from build123d import *

# Parameters (mm, degrees)
EXTRUDE_1_DEPTH = 815
SHELL_1_T       = -3


with BuildPart() as part:
    # Эскиз1 → Бобышка-Вытянуть1 (new, symmetric)
    with BuildSketch(Plane.XY):
        with BuildLine():
            Line((-25, -30), (25, -30))
            ThreePointArc((25, -30), (28.535533906, -28.535533906), (30, -25))
            Line((30, -25), (30, 25))
            ThreePointArc((30, 25), (28.535533906, 28.535533906), (25, 30))
            Line((25, 30), (-25, 30))
            ThreePointArc((-25, 30), (-28.535533906, 28.535533906), (-30, 25))
            Line((-30, 25), (-30, -25))
            ThreePointArc((-30, -25), (-28.535533906, -28.535533906), (-25, -30))
        make_face()
    extrude(amount=EXTRUDE_1_DEPTH, both=True)

    # Оболочка1
    shell_1_openings = [part.faces().sort_by_distance(p)[0] for p in [
        (0, 0, 815),
        (0, 0, -815),
    ]]
    offset(amount=SHELL_1_T, openings=shell_1_openings, kind=Kind.INTERSECTION)


solid = part.part
Input: part model. Units: mm. Frame: model coordinates. A direction names the side the tool comes from. Give positions to 0.01 mm unless a question says otherwise; leave off trailing zeros. Write each loop counter-clockwise with the first axis right and the second up, starting at its lowest first coordinate (ties: lowest second). Pieces come first, ordered by that corner, then holes. Notation, with made-up numbers: (-0.5, -3) -> (50.5, -3) arc R12 ccw to (50.5, 4) -> close; hole circle Ø8 at (48, 45.25). An arc over 180 degrees is marked (long way). Use one line per item in the form item = value. Start each with the question number.
1) Section query A-A on x = 5. Return the cut outline in (y, z), then the cut area to 3 significant figures.
2) Set-up query: faces 4 (the flat face through (27, 0, 11)), 5 (the flat face through (-2, -29, -815)). Return all of +Z, -Z, +X, -X, +Y, -Y with unobstructed straight access to the full face (end or side cutting, diameter ignored); none if empty.
3) Ray query, probe 1 along Y at (x, z) = (-23, 401); probe 2 along Y at (x, z) = (25.5, -297). Return the intervals inside material, ascending. Write a range as from..to.
4) Section query C-C on z = -130. Return the cut outline in (x, y).
5) Draft query along Y for faces 1 (the flat face through (-27, 0, 11)), 2 (the flat face through (-2, -29, 815)), 3 (the flat face through (0, -30, 11)). Return one class per face: pulls with the +Y half, pulls with the -Y half, needs draft (parallel to the pull), parting line crosses it, or undercut.
Outcome:
q1.outline = (-30, -815) -> (-27, -815) -> (-27, 815) -> (-30, 815) -> close; (27, -815) -> (30, -815) -> (30, 815) -> (27, 815) -> close
q1.area = 9,780 mm^2
q2.face_4 = +Z, -Z
q2.face_5 = -Z, +X, -X, +Y, -Y
q3.probe_1 = -30..-27, 27..30
q3.probe_2 = -29.97..-26.94, 26.94..29.97
q4.outline = (-30, -25) arc R5 ccw to (-25, -30) -> (25, -30) arc R5 ccw to (30, -25) -> (30, 25) arc R5 ccw to (25, 30) -> (-25, 30) arc R5 ccw to (-30, 25) -> close; hole (-27, -25) arc R2 ccw to (-25, -27) -> (25, -27) arc R2 ccw to (27, -25) -> (27, 25) arc R2 ccw to (25, 27) -> (-25, 27) arc R2 ccw to (-27, 25) -> close
q5.face_1 = undercut
q5.face_2 = needs draft
q5.face_3 = pulls with the -Y half
